Autodesk Inventor part; units mm, degrees
ref_plane "YZ Plane" through (0, 0, 0) normal (1, 0, 0) x (0, 1, 0)
ref_plane "XZ Plane" through (0, 0, 0) normal (0, 1, 0) x (-1, 0, 0)
ref_plane "XY Plane" through (0, 0, 0) normal (0, 0, 1) x (1, 0, 0)
sketch "Esquisse1" plane through (0, 0, 0) normal (0, 1, 0) x (-1, 0, 0)
  line L0 (0, 0) -> (0, -8)
  line L1 (0, 0) -> (8, 0)
  line L2 (8, 0) -> (8, -29)
  line L3 (8, -29) -> (50, -29)
  line L4 (50, -29) -> (50, 0)
  line L5 (0, -8) -> (4, -8)
  line L6 (4, -8) -> (4, -50)
  line L7 (50, 0) -> (58, 0)
  line L8 (58, 0) -> (58, -34)
  line L9 (58, -34) -> (4, -50)
  dimension "d0" = 8
  dimension "d1" = 29
  dimension "d2" = 42
  dimension "d3" = 8
  dimension "d4" = 42
  dimension "d5" = 8
  dimension "d6" = 34
  dimension "d11" = 4
  dimension "d12" = 29
extrude "Extrusion1" add sketch "Esquisse1" along normal blind 20
sketch "Esquisse2" plane through (-58, 0, 0) normal (0, 0, 1) x (1, 0, 0)
  line L0 (0, 20) -> (8, 20)
  line L1 (0, 0) -> (8, 0)
  line L2 (0, 0) -> (0, 20)
  point P0 (58, 0)
  point P1 (4, 15)
  point P2 (4, 5)
  dimension "d15" = 10
  dimension "d17" = 5
  dimension "d18" = 4
  dimension "d19" = 4
hole "Perçage1" at (-54, 15, 0) at (-54, 5, 0) direction (0, 0, -1) diameter 4 depth 10 tip angle 118
sketch "Esquisse3" plane through (-8, 0, 0) normal (0, 0, 1) x (1, 0, 0)
  line L0 (0, 20) -> (8, 20)
  line L1 (8, 0) -> (8, 20)
  point P0 (4, 15)
  point P1 (4, 5)
  dimension "d27" = 10
  dimension "d28" = 5
  dimension "d29" = 4
  dimension "d30" = 4
hole "Perçage2" at (-4, 15, 0) at (-4, 5, 0) direction (0, 0, -1) diameter 4 depth 10 tip angle 118
sketch "Esquisse4" plane through (-4, 0, -8) normal (1, 0, 0) x (0, 0, -1)
  line L0 (42, 5) -> (27.5, 5)
  line L1 (27.5, 5) -> (27.5, 15)
  line L2 (27.5, 15) -> (42, 15)
  line L3 (42, 15) -> (42, 5)
  line L4 (0, 0) -> (42, 0)
  line L5 (42, 0) -> (42, 20)
  point P0 (-8, 0)
  dimension "d38" = 10
  dimension "d39" = 14.5
  dimension "d40" = 5
  dimension "d41" = 0
extrude "Extrusion2" cut sketch "Esquisse4" against normal blind 100
sketch "Esquisse5" plane through (-4, 15, -50) normal (0, -1, 0) x (1, 0, 0)
  line L0 (0, 42) -> (0, 0)
  line L1 (-4, 21) -> (0, 21)
  line L2 (0, 21) -> (0, 0)
  line L3 (0, 0) -> (-4, 0)
  line L4 (-4, 0) -> (-4, 21)
  point P0 (4, 50)
extrude "Extrusion3" add sketch "Esquisse5" along normal blind 10
sketch "Esquisse6" plane through (-4, 0, -8) normal (1, 0, 0) x (0, 0, -1)
  line L0 (11, 5.5) -> (17, 5.5)
  line L1 (17, 5.5) -> (17, 14.5)
  line L2 (17, 14.5) -> (11, 14.5)
  line L3 (11, 14.5) -> (11, 5.5)
  line L4 (-8, 0) -> (-8, 20)
  line L5 (21, 20) -> (-8, 20)
  dimension "d49" = 19
  dimension "d50" = 25
  dimension "d51" = 9
  dimension "d52" = 5.5
extrude "Extrusion4" cut sketch "Esquisse6" against normal blind 10
sketch "Esquisse7" plane through (-4, 0, -8) normal (1, 0, 0) x (0, 0, -1)
  line L0 (-8, 0) -> (-8, 20)
  line L1 (42, 15) -> (42, 5)
  line L2 (21, 0) -> (-8, 0)
  line L3 (42, 0) -> (26, 0)
  point P0 (1.5, 10)
  point P1 (32.5, 10)
  dimension "d55" = 9.5
  dimension "d56" = 9.5
  dimension "d57" = 10
  dimension "d58" = 10
hole "Perçage3" at (-4, 10, -9.5) at (-4, 10, -40.5) direction (-1, 0, 0) diameter 3 depth 20 tip angle 118
chamfer "Chanfrein2" distance 2 angle 45 1 edges at (-8, 10, -8)
sketch "Esquisse8" plane through (-8, 0, -29) normal (-1, 0, 0) x (0, 0, 1)
  line L0 (4, 14.5) -> (4, 5.5)
  line L1 (21, 0) -> (-21, 0)
  line L2 (4, 5.5) -> (10, 5.5)
  line L3 (10, 5.5) -> (10, 0)
  line L4 (10, 0) -> (4, 0)
  line L5 (4, 0) -> (4, 5.5)
  point P0 (29, 0)
  dimension "d69" = 6
extrude "Extrusion5" cut sketch "Esquisse8" against normal blind 2
chamfer "Chanfrein3" distance 4 angle 45 1 edges at (-8, 10, -50)
properties part number "supportservopetitrobot"
Source: CAD feature listing. Evaluate the final solid. Frame: model axes, mm. A direction names the side the tool comes from. Give positions to 0.01 mm unless a question says otherwise; leave off trailing zeros. Write each loop counter-clockwise with the first axis right and the second up, starting at its lowest first coordinate (ties: lowest second). Pieces come first, ordered by that corner, then holes. Notation, with made-up numbers: M 44,64 L 79,64 A31 cw 79,97 Z; hole C 75,-34 d8. An arc over 180 degrees is marked long. Return JSON: item names as keys, results as strings. Group by question number.
1) First-contact query: pin 1 Ø3 at (x, z) = (-7, -21.5) entering from -Y; pin 2 Ø2 at (x, y) = (-34.5, 7) entering from +Z; pin 3 Ø6 at (y, z) = (10, -15.5) entering from +X; pin 4 Ø10 at (x, y) = (-47, 12.5) entering from -Z. Flat tips, straight axial feed; report the tip coordinate or a pass-through.
2) Draft query along Z for faces 5 (the face through (-21, 5, -40)), 6 (the face through (-4.792, 15.017, -10.726)), 7 (the face through (-6, 9, -25)). Return one class per face: released by +Z, released by -Z, zero draft, split by the parting line, or undercut.
3) Set-up query: faces 1 (the face through (-29, 10, -29)), 2 (the face through (-5, 10.9, -8.3)), 3 (the face through (-6, 3, -22)), 4 (the face through (-8, 9, -42)). Return all of +Z, -Z, +X, -X, +Y, -Y with unobstructed straight access to the full face (end or side cutting, diameter ignored); none if empty.
4) Cut plane D-D, the plane x = -45.5. Output: boundary loops of the cut face in (y, z), then the cut area to 3 significant figures.
5) Ray query, L1, parallel to X at y = 5, z = -7; L2, parallel to Y at x = -54, z = -4; L3, parallel to X at y = 16.5, z = -28.5. Return the intervals inside material, ascending.
6) Cut plane C-C, the plane z = -21. Output: boundary loops of the cut face in (x, y).
7) Cut plane A-A, the plane z = -27.5. Output: boundary loops of the cut face in (x, y), then the cut area to 3 significant figures.
8) Cut plane B-B, the plane y = 18.5. Output: boundary loops of the cut face in (x, z).
Data:
{
 "1": {"pin 1": "stops at y = 0", "pin 2": "stops at z = -29", "pin 3": "stops at x = -4", "pin 4": "stops at z = -38.54"},
 "2": {"face 5": "zero draft", "face 6": "released by +Z", "face 7": "undercut"},
 "3": {"face 1": "+Z, +Y, -Y", "face 2": "+X", "face 3": "-Y", "face 4": "-Z, -X"},
 "4": {"outline": "M 0,-37.7 L 5,-37.7 L 5,-35.5 L 15,-35.5 L 15,-37.7 L 20,-37.7 L 20,-29 L 0,-29 Z", "area": "152 mm²"},
 "5": {"L1": "x = -58 to -56, -52 to -50, -8 to -6, -2 to 0", "L2": "y = 0 to 3, 7 to 13, 17 to 20", "L3": "x = -58 to -50, -8 to -4"},
 "6": {"outline": "M -58,0 L -50,0 L -50,20 L -58,20 Z; M -8,14.5 L -4,14.5 L -4,20 L -8,20 Z; M -6,0 L -4,0 L -4,5.5 L -6,5.5 Z"},
 "7": {"outline": "M -58,0 L -50,0 L -50,20 L -58,20 Z; M -8,0 L -4,0 L -4,20 L -8,20 Z", "area": "240 mm²"},
 "8": {"outline": "M -58,-34 L -4,-50 L -4,-8 L 0,-8 L 0,0 L -8,0 L -8,-29 L -50,-29 L -50,0 L -58,0 Z"}
}
